The model under review builds one solid part; all positions refer to its coordinate system, in mm. A direction names the side the tool comes from. Round coordinates to 2 decimals unless told otherwise and drop trailing zeros. Write each loop counter-clockwise with the first axis right and the second up, starting at its lowest first coordinate (ties: lowest second). Pieces come first, ordered by that corner, then holes. Notation, with made-up numbers: (76, -35.75) - (104, -35.75) arc R8 cw to (104, -26.75) - close; hole circle Ø8 at (-15.5, -14). An arc over 180 degrees is marked (long way). Return JSON: item names as keys, results as strings.
from build123d import *
from build123d.topology import SkipClean

# Parameters (mm, degrees)
SALIENTE_EXTRUIR1_DEPTH    = 200
CROQUIS2_W                 = 2.5
CROQUIS2_H                 = 180
SALIENTE_EXTRUIR2_DEPTH    = 42.5
CROQUIS3_R                 = 5.5
CORTAR_EXTRUIR1_DEPTH      = 4
CROQUIS4_R                 = 3.75
CORTAR_EXTRUIR2_DEPTH      = 4
CROQUIS7_W                 = 12.1
CROQUIS7_H                 = 10.75
CORTAR_EXTRUIR3_DEPTH      = 4
REDONDEO1_R                = 0.3
CROQUIS8_R                 = 1.425
SALIENTE_EXTRUIR3_DEPTH    = 5
SIMETR_A2_COPY_1_SKETCH_R  = 1.425
SIMETR_A2_COPY_1_DEPTH     = 5
REDONDEO4_START            = 29.9999999
REDONDEO4_OUTLINE_R        = 1.425
REDONDEO4_DEPTH            = 10.0000001
REDONDEO4_2_OUTLINE_W      = 10
REDONDEO4_2_OUTLINE_H      = 9.000004552
REDONDEO4_2_OUTLINE_H_2    = 9.000004551
REDONDEO5_START            = 29.9999999
REDONDEO5_OUTLINE_R        = 1.425
REDONDEO5_DEPTH            = 10.0000001
REDONDEO5_2_OUTLINE_W      = 10
REDONDEO5_2_OUTLINE_H      = 9.000004551
REDONDEO5_2_OUTLINE_H_2    = 9.000004552
CROQUIS9_W                 = 67
CROQUIS9_H                 = 37
SALIENTE_EXTRUIR4_DEPTH    = 20
CORTAR_EXTRUIR5_DEPTH      = 1
CORTAR_EXTRUIR5_DEPTH_BACK = 66
CROQUIS11_W                = 69.586098965
CROQUIS11_H                = 38.970086607
CORTAR_EXTRUIR6_DEPTH      = 9
CROQUIS12_W                = 37
CROQUIS12_H                = 10.997736301
SALIENTE_EXTRUIR5_DEPTH    = 0.7
CROQUIS14_W                = 66
CROQUIS14_H                = 7.054690465
CORTAR_EXTRUIR7_DEPTH      = 7.7


with BuildPart() as part:
    # Croquis1 → Saliente-Extruir1 (new body)
    with BuildSketch(Plane(origin=(0, 0, 0), x_dir=(0, 0, -1), z_dir=(1, 0, 0))):
        Polygon((90, 9.273962115), (90, 0), (-90, 0), (-90, 9.273962115), (-88.2, 7.766551311), (-88.2, 2.5), (88.2, 2.5), (88.2, 7.766551311), align=None)
    extrude(amount=SALIENTE_EXTRUIR1_DEPTH)

    # Croquis2 → Saliente-Extruir2 (add)
    with BuildSketch(Plane(origin=(0, 2.5, 0), x_dir=(1, 0, 0), z_dir=(0, 1, 0))):
        with Locations((198.75, 0)):
            Rectangle(CROQUIS2_W, CROQUIS2_H)
        with Locations((1.25, 0)):
            Rectangle(CROQUIS2_W, CROQUIS2_H)
    extrude(amount=SALIENTE_EXTRUIR2_DEPTH)

    # Croquis3 → Cortar-Extruir1 (cut)
    with BuildSketch(Plane(origin=(200, 0, 0), x_dir=(0, 0, -1), z_dir=(1, 0, 0))):
        with Locations((75, 15)):
            Circle(CROQUIS3_R)
    extrude(amount=-CORTAR_EXTRUIR1_DEPTH, mode=Mode.SUBTRACT)

    # Croquis4 → Cortar-Extruir2 (cut)
    with BuildSketch(Plane(origin=(200, 0, 0), x_dir=(0, 0, -1), z_dir=(1, 0, 0))):
        with Locations((55, 15)):
            Circle(CROQUIS4_R)
    extrude(amount=-CORTAR_EXTRUIR2_DEPTH, mode=Mode.SUBTRACT)

    # Croquis7 → Cortar-Extruir3 (cut)
    with BuildSketch(Plane(origin=(200, 0, 0), x_dir=(0, 0, -1), z_dir=(1, 0, 0))):
        with Locations((35, 15)):
            Rectangle(CROQUIS7_W, CROQUIS7_H)
    extrude(amount=-CORTAR_EXTRUIR3_DEPTH, mode=Mode.SUBTRACT)

    # Redondeo1
    redondeo1_edges = [part.edges().sort_by_distance(p)[0] for p in [
        (198.75, 20.375, -41.05),
        (198.75, 9.625, -41.05),
        (198.75, 9.625, -28.95),
        (198.75, 20.375, -28.95),
    ]]
    fillet(redondeo1_edges, radius=REDONDEO1_R)

    # Croquis8 → Saliente-Extruir3 (add)
    with BuildSketch(Plane(origin=(0, 45, 0), x_dir=(1, 0, 0), z_dir=(0, 1, 0))):
        with BuildLine():
            Line((192, -74.506703602), (197.5, -74.506703602))
            Line((197.5, -74.506703602), (197.5, -83.506703602))
            Line((197.5, -83.506703602), (192, -83.506703602))
            ThreePointArc((192, -83.506703602), (187.5, -79.006703602), (192, -74.506703602))
        make_face()
        with Locations(Location((192, -79.006703602, 0), (0, 0, 270))):
            Circle(CROQUIS8_R, mode=Mode.SUBTRACT)
    saliente_extruir3 = extrude(amount=-SALIENTE_EXTRUIR3_DEPTH)

    # Simetría1: Saliente-Extruir3 across plane
    add(saliente_extruir3.mirror(Plane.XY))

    # Simetría2: Saliente-Extruir3 across plane
    add(saliente_extruir3.mirror(Plane(origin=(100, 0, 0), x_dir=(0, 0, 1), z_dir=(1, 0, 0))))

    # Simetría2 copy 1 sketch → Simetría2 copy 1 (add)
    with BuildSketch(Plane(origin=(200, 45, 0), x_dir=(-1, 0, 0), z_dir=(0, 1, 0))):
        with BuildLine():
            Line((192, -74.506703602), (197.5, -74.506703602))
            Line((197.5, -74.506703602), (197.5, -83.506703602))
            Line((197.5, -83.506703602), (192, -83.506703602))
            ThreePointArc((192, -83.506703602), (187.5, -79.006703602), (192, -74.506703602))
        make_face()
        with Locations(Location((192, -79.006703602, 0), (0, 0, 270))):
            Circle(SIMETR_A2_COPY_1_SKETCH_R, mode=Mode.SUBTRACT)
    extrude(amount=-SIMETR_A2_COPY_1_DEPTH)

    # Redondeo4: read off the stored shape, not the designer's step
    # Redondeo4 outline → Redondeo4 (add)
    # profile 1 of 2: a face of its own
    with SkipClean():  # the faces are left unmerged after this step: merging them gives an invalid solid
        with BuildSketch(Plane(origin=(0, 0, 0), x_dir=(1, 0, 0), z_dir=(0, 1, 0)).offset(REDONDEO4_START)):
            with BuildLine():
                Line((197.5, -74.506703602), (192, -74.506703602))
                ThreePointArc((192, -74.506703602), (187.5, -79.006703602), (192, -83.506703602))
                Line((192, -83.506703602), (197.5, -83.506703602))
                Line((197.5, -83.506703602), (197.5, -74.506703602))
            make_face()
            with Locations((192, -79.006703602)):
                Circle(REDONDEO4_OUTLINE_R, mode=Mode.SUBTRACT)
        # profile 2 of 2: a face of its own
        with BuildSketch(Plane(origin=(0, 0, 0), x_dir=(1, 0, 0), z_dir=(0, 1, 0)).offset(REDONDEO4_START)):
            with BuildLine():
                Line((192, 74.506703602), (197.5, 74.506703602))
                Line((197.5, 74.506703602), (197.5, 83.506703602))
                Line((197.5, 83.506703602), (192, 83.506703602))
                ThreePointArc((192, 83.506703602), (187.5, 79.006703602), (192, 74.506703602))
            make_face()
            with Locations((192, 79.006703602)):
                Circle(REDONDEO4_OUTLINE_R, mode=Mode.SUBTRACT)
        extrude(amount=REDONDEO4_DEPTH)
    add(part.part.scale(1), mode=Mode.REPLACE)  # the faces are merged on a copy

    # Redondeo4 2 outline → Redondeo4 2 (revolve, cut)
    with BuildSketch(Plane(origin=(187.5, 30, 0), x_dir=(1, 0, 0), z_dir=(0, -1, 0))):
        with Locations((5, -79.006704338)):
            Rectangle(REDONDEO4_2_OUTLINE_W, REDONDEO4_2_OUTLINE_H)
        with Locations((5, 79.006702866)):
            Rectangle(REDONDEO4_2_OUTLINE_W, REDONDEO4_2_OUTLINE_H_2)
    revolve(axis=Axis((187.5, 30, 0), (0, 0, 1)), mode=Mode.SUBTRACT)

    # Redondeo5: read off the stored shape, not the designer's step
    # Redondeo5 outline → Redondeo5 (add)
    # profile 1 of 2: a face of its own
    with BuildSketch(Plane(origin=(0, 0, 0), x_dir=(1, 0, 0), z_dir=(0, 1, 0)).offset(REDONDEO5_START)):
        with BuildLine():
            Line((2.5, 83.506703602), (2.5, 74.506703602))
            Line((2.5, 74.506703602), (8, 74.506703602))
            ThreePointArc((8, 74.506703602), (12.5, 79.006703602), (8, 83.506703602))
            Line((8, 83.506703602), (2.5, 83.506703602))
        make_face()
        with Locations((8, 79.006703602)):
            Circle(REDONDEO5_OUTLINE_R, mode=Mode.SUBTRACT)
    # profile 2 of 2: a face of its own
    with BuildSketch(Plane(origin=(0, 0, 0), x_dir=(1, 0, 0), z_dir=(0, 1, 0)).offset(REDONDEO5_START)):
        with BuildLine():
            Line((8, -74.506703602), (2.5, -74.506703602))
            Line((2.5, -74.506703602), (2.5, -83.506703602))
            Line((2.5, -83.506703602), (8, -83.506703602))
            ThreePointArc((8, -83.506703602), (12.5, -79.006703602), (8, -74.506703602))
        make_face()
        with Locations((8, -79.006703602)):
            Circle(REDONDEO5_OUTLINE_R, mode=Mode.SUBTRACT)
    extrude(amount=REDONDEO5_DEPTH)

    # Redondeo5 2 outline → Redondeo5 2 (revolve, cut)
    with BuildSketch(Plane(origin=(12.5, 30, 0), x_dir=(1, 0, 0), z_dir=(0, -1, 0))):
        with Locations((5, -79.006702866)):
            Rectangle(REDONDEO5_2_OUTLINE_W, REDONDEO5_2_OUTLINE_H)
        with Locations((5, 79.006704338)):
            Rectangle(REDONDEO5_2_OUTLINE_W, REDONDEO5_2_OUTLINE_H_2)
    revolve(axis=Axis((12.5, 30, 0), (0, 0, 1)), mode=Mode.SUBTRACT)

    # Croquis9 → Saliente-Extruir4 (add)
    with BuildSketch(Plane(origin=(0, 2.5, 0), x_dir=(1, 0, 0), z_dir=(0, 1, 0))):
        with Locations((157.239750521, -6.353396278)):
            Rectangle(CROQUIS9_W, CROQUIS9_H)
    extrude(amount=SALIENTE_EXTRUIR4_DEPTH)

    # Croquis10 → Cortar-Extruir5 (cut, two sides: drawn at the far end of the back side and taken through both)
    with BuildSketch(Plane(origin=(190.739750521, 0, 0), x_dir=(0, 0, -1), z_dir=(1, 0, 0)).offset(-CORTAR_EXTRUIR5_DEPTH_BACK)):
        with BuildLine():
            ThreePointArc((-6.420068532, 16.930863921), (-24.676853259, 13.247289401), (-6.420068532, 9.563714882))
            ThreePointArc((-6.420068532, 9.563714882), (11.836716195, 13.247289401), (-6.420068532, 16.930863921))
        make_face()
    extrude(amount=CORTAR_EXTRUIR5_DEPTH + CORTAR_EXTRUIR5_DEPTH_BACK, mode=Mode.SUBTRACT)

    # Croquis11 → Cortar-Extruir6 (cut)
    with BuildSketch(Plane(origin=(0, 22.5, 0), x_dir=(1, 0, 0), z_dir=(0, 1, 0))):
        with Locations((157.239750521, -6.353396279)):
            Rectangle(CROQUIS11_W, CROQUIS11_H)
    extrude(amount=-CORTAR_EXTRUIR6_DEPTH, mode=Mode.SUBTRACT)

    # Croquis12 → Saliente-Extruir5 (add)
    with BuildSketch(Plane(origin=(190.739750521, 0, 0), x_dir=(0, 0, -1), z_dir=(1, 0, 0))):
        with Locations((-6.353396278, 7.998868151)):
            Rectangle(CROQUIS12_W, CROQUIS12_H)
    extrude(amount=SALIENTE_EXTRUIR5_DEPTH)

    # Croquis14 → Cortar-Extruir7 (cut)
    with BuildSketch(Plane(origin=(0, 13.497736301, 0), x_dir=(1, 0, 0), z_dir=(0, 1, 0))):
        with Locations((157.739750521, -6.420068533)):
            Rectangle(CROQUIS14_W, CROQUIS14_H)
    extrude(amount=-CORTAR_EXTRUIR7_DEPTH, mode=Mode.SUBTRACT)


solid = part.part
(1) Add section D-D (z = -24.5). Write out the cut boundary in (x, y), plus the area to 4 significant figures.
Filled in:
{"outline": "(0, 0) - (200, 0) - (200, 45) - (197.5, 45) - (197.5, 2.5) - (2.5, 2.5) - (2.5, 45) - (0, 45) - close", "area": "712.5 mm2"}
(2) Wall thickness on line 1 (Z direction, x = 192, y = 39.35); line 2 (X direction, y = 15, z = 67.5); line 3 (Y direction, x = 198, z = -55): over which ranges is each line inside the solid? List them lowest first.
Filled in:
{"line 1": "z = -83.51 to -80.43, -77.58 to -74.51, 74.51 to 77.58, 80.43 to 83.51", "line 2": "x = 0 to 2.5, 197.5 to 200", "line 3": "y = 0 to 11.25, 18.75 to 45"}
(3) Add section C-C (x = 78.5). Write out the cut boundary in (y, z), plus the area to 3 significant figures.
Filled in:
{"outline": "(0, -90) - (9.27, -90) - (7.77, -88.2) - (2.5, -88.2) - (2.5, 88.2) - (7.77, 88.2) - (9.27, 90) - (0, 90) - close", "area": "472 mm2"}
(4) Clearance check with flat-ended pins moving along their axes: pin 1 Ø2.5 at (x, z) = (192, -79.01) entering from -Y; pin 2 Ø4.5 at (x, y) = (194, 35.5) entering from +Z; pin 3 Ø7 at (y, z) = (15, -55) entering from +X; pin 4 Ø1.7 at (x, z) = (192, -79.01) entering from +Y. State where each tip first meets the part, or that it passes through.
Filled in:
{"pin 1": "stops at y = 0", "pin 2": "stops at z = 83.51", "pin 3": "stops at x = 2.5", "pin 4": "stops at y = 2.5"}
(5) Add section A-A (y = 23). Write out the cut boundary in (x, z), plus the area to 3 significant figures.
Filled in:
{"outline": "(0, -90) - (2.5, -90) - (2.5, 90) - (0, 90) - close; (197.5, -90) - (200, -90) - (200, 90) - (197.5, 90) - close", "area": "900 mm2"}
(6) Add section B-B (z = -55). Write out the cut boundary in (x, y), plus the area to 3 significant figures.
Filled in:
{"outline": "(0, 0) - (200, 0) - (200, 11.25) - (197.5, 11.25) - (197.5, 2.5) - (2.5, 2.5) - (2.5, 45) - (0, 45) - close; (197.5, 18.75) - (200, 18.75) - (200, 45) - (197.5, 45) - close", "area": "694 mm2"}
(7) For faces 1 (the flat face through (157, 8, 24.853)), 2 (the flat face through (5, 41, 83.507)), 3 (the cylindrical face through (198.768, 13.564, -58.464)), list the 3-axis set-ups (+Z, -Z, +X, -X, +Y, -Y) from which the entire face can be reached by the end or side of a thin tool; tool diameter is ignored.
Filled in:
{"face 1": "+Y", "face 2": "+Z, +Y", "face 3": "+X"}
(8) Mouldability with a two-part tool opening along X and no side actions: class faces 4 (the flat face through (2, 45, -1)), 5 (the flat face through (0, 23, -1)), 6 (the flat face through (99, 2.5, 1)) as released by +X, released by -X, zero draft, split by the parting line, or undercut.
Filled in:
{"face 4": "zero draft", "face 5": "released by -X", "face 6": "undercut"}
